from build123d import *

# Parameters (mm, degrees)
F1_ANGLE    = 180
F2_R        = 5
F3_R        = 1
F4_T2_ANGLE = 242.2675380927


# Not quite as in the source:
# - a fillet or chamfer that OpenCascade refuses, or shapes differently, is made with other operations: its cross-section is extruded or revolved along the edge and cut away or added


with BuildPart() as f1:
    # F0 (on Front) → F1 (revolve)
    with BuildSketch(Plane.XZ):
        Polygon((14, -25), (4.157225346, -15.157225346), (7.7397023427, -25), (7.7397023427, -30), (14, -30), align=None)
    revolve(axis=Axis((0, 0, 0), (0, 0, -1)), revolution_arc=F1_ANGLE)

    # F2
    f2_edges = [f1.edges().sort_by_distance(p)[0] for p in [
        (0, -14, -25),
    ]]
    fillet(f2_edges, radius=F2_R)

    # F3
    f3_edges = [f1.edges().sort_by_distance(p)[0] for p in [
        (0, -14, -30),
        (0, -7.739702, -30),
    ]]
    fillet(f3_edges, radius=F3_R)

    # F4: fillet of radius 0.2 on 1 edges, made by hand

    # F4_s1 → F4_t2 (revolve, cut)
    with BuildSketch(Plane(origin=(0, 0, 0), x_dir=(0, 0, 1), z_dir=(-0.5170379067, 0.8559625009, 0))):
        with BuildLine():
            ThreePointArc((-15.7951358602, 4.7951358602), (-15.7678789273, 4.5462545823), (-16.0049612451, 4.4657759798))
            Line((-16.0049612451, 4.4657759798), (-15.157225346, 4.157225346))
            Line((-15.157225346, 4.157225346), (-15.7951358602, 4.7951358602))
        make_face()
    revolve(axis=Axis((0, 0, -15.157225346), (0, 0, -1)), revolution_arc=F4_T2_ANGLE, mode=Mode.SUBTRACT)


solid = f1.part
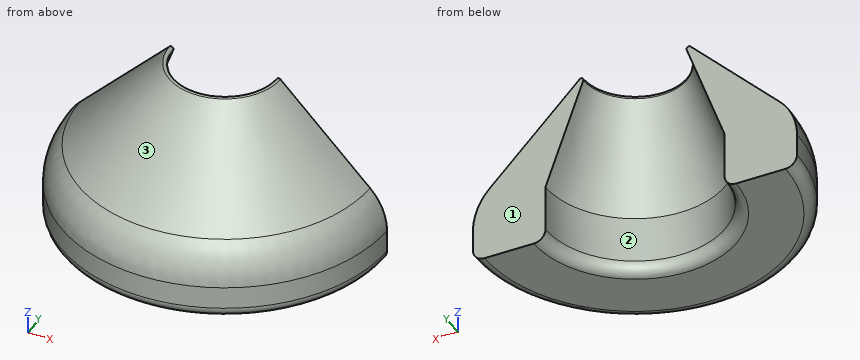
Source: CAD feature listing. Evaluate the final solid. Frame: model axes, mm. Face numbers are marked on the shaded views. Round coordinates to 2 decimals unless told otherwise and drop trailing zeros. Loops run counter-clockwise (first coordinate to the right, second up) from the corner with the lowest first, then second, coordinate; pieces in that order, holes last. Notation, with made-up numbers: M -27.75,48 L -17.75,48 A24 cw -17.75,80 Z; hole C 44,-19 d8. An arc over 180 degrees is marked long. Answer as CSV lines item,"result".
Q1. Cut plane A-A (z = -22). Return the cut outline in (x, y).
Verdict:
outline,"M -11,0 A11 ccw 11,0 L 6.65,0 A6.65 cw -6.65,0 Z"
Q2. Contact query for flat-ended pins moving along their axis: pin 1 (1.5 mm diameter, centred on y = -6.5, z = -19, fed in from +X); pin 2 (2 mm diameter, centred on x = -3, y = -4, fed in from +Z); pin 3 (1 mm diameter, centred on x = -10.5, y = -6, fed in from +Z); pin 4 (1.5 mm diameter, centred on x = -4, y = -7, fed in from +Z). Output: stop coordinate, or through.
Verdict:
pin 1,"stops at x = 6.11"
pin 2,"stops at z = -15.74"
pin 3,"stops at z = -22.59"
pin 4,"stops at z = -18.31"
Q3. Pull-direction query (X, two-part tool) for the marked faces 1, 2 and 3; classes: +X half, -X half, draft (parallel to the pull), parting line (faces both ways), or undercut.
Verdict:
face 1,"draft"
face 2,"undercut"
face 3,"parting line"
Q4. Cut plane B-B (z = -20). Return the cut outline in (x, y).
Verdict:
outline,"M -9,0 A9 ccw 9,0 L 5.92,0 A5.92 cw -5.92,0 Z"
Q5. Line query: line 1 along Y through (x, z) = (0.25, -27.75); line 2 along X through (y, z) = (-3.5, -25); line 3 along X through (y, z) = (-4, -25.5). Output: solid intervals per line, ascending.
Verdict:
line 1,"y = -14 to -7.74"
line 2,"x = -13.09 to -6.9, 6.9 to 13.09"
line 3,"x = -13.15 to -6.63, 6.63 to 13.15"
